from build123d import *

# Parameters (mm, degrees)
SKETCH_1_W                         = 130
SKETCH_1_H                         = 22
ARM_WEB_L130_W22_T6_DEPTH          = 6
SKETCH_2_R                         = 14
SPLIT_CLAMP_HUB_DEPTH              = 12
SKETCH_3_R                         = 16
WRIST_END_R16_DEPTH                = 6
SHAFT_D5P2_AND_WRIST_M3_DEPTH      = 148.363496158
SHAFT_D5P2_AND_WRIST_M3_DEPTH_BACK = 148.363496158
SKETCH_4_R                         = 2.6
SKETCH_4_R_2                       = 1.7
CLAMP_SPLIT_1P2_DEPTH              = 148.363496158
CLAMP_SPLIT_1P2_DEPTH_BACK         = 148.363496158
SKETCH_5_W                         = 1.2
SKETCH_5_H                         = 12.8
CLAMP_CROSSBOLT_M3_DEPTH           = 148.363496158
CLAMP_CROSSBOLT_M3_DEPTH_BACK      = 148.363496158
SKETCH_6_R                         = 1.7


with BuildPart() as part:
    # 草图1 → Arm_web_L130_W22_T6 (new body)
    with BuildSketch(Plane.XY):
        with Locations((65, 0)):
            Rectangle(SKETCH_1_W, SKETCH_1_H)
    extrude(amount=ARM_WEB_L130_W22_T6_DEPTH)

    # 草图2 → Split_clamp_hub (add)
    with BuildSketch(Plane.XY):
        with Locations(Location((0, 0, 0), (0, 0, 308.213210702))):
            Circle(SKETCH_2_R)
    extrude(amount=SPLIT_CLAMP_HUB_DEPTH)

    # 草图3 → Wrist_end_R16 (add)
    with BuildSketch(Plane.XY):
        with Locations((130, 0)):
            Circle(SKETCH_3_R)
    extrude(amount=WRIST_END_R16_DEPTH)

    # 草图4 → Shaft_D5p2_and_wrist_M3 (cut, two sides: drawn at the far end of the back side and taken through both)
    with BuildSketch(Plane.XY.offset(-SHAFT_D5P2_AND_WRIST_M3_DEPTH_BACK)):
        Circle(SKETCH_4_R)
        with Locations((124, 0)):
            Circle(SKETCH_4_R_2)
        with Locations((136, 0)):
            Circle(SKETCH_4_R_2)
    extrude(amount=SHAFT_D5P2_AND_WRIST_M3_DEPTH + SHAFT_D5P2_AND_WRIST_M3_DEPTH_BACK, mode=Mode.SUBTRACT)

    # 草图5 → Clamp_split_1p2 (cut, two sides: drawn at the far end of the back side and taken through both)
    with BuildSketch(Plane.XY.offset(-CLAMP_SPLIT_1P2_DEPTH_BACK)):
        with Locations((0, 8.6)):
            Rectangle(SKETCH_5_W, SKETCH_5_H)
    extrude(amount=CLAMP_SPLIT_1P2_DEPTH + CLAMP_SPLIT_1P2_DEPTH_BACK, mode=Mode.SUBTRACT)

    # 草图6 → Clamp_crossbolt_M3 (cut, two sides: drawn at the far end of the back side and taken through both)
    with BuildSketch(Plane(origin=(0, 0, 0), x_dir=(0, 0, -1), z_dir=(1, 0, 0)).offset(-CLAMP_CROSSBOLT_M3_DEPTH_BACK)):
        with Locations((-8.5, 9)):
            Circle(SKETCH_6_R)
    extrude(amount=CLAMP_CROSSBOLT_M3_DEPTH + CLAMP_CROSSBOLT_M3_DEPTH_BACK, mode=Mode.SUBTRACT)


solid = part.part
CAD build for the part. Positions are in the model's coordinates, mm. A direction names the side the tool comes from. Round coordinates to 2 decimals unless told otherwise and drop trailing zeros. Order: outer loops, then holes, each group sorted by start corner. A loop starts at its lowest first (then second) coordinate and runs counter-clockwise, first axis right, second up. Notation, with made-up numbers: (-1.75, 53.25) - (13.25, 53.25) arc R26 cw to (13.25, 83.25) - close; hole circle Ø10 at (68, 67.25). An arc over 180 degrees is marked (long way). Return JSON: item names as keys, results as strings.
(1) Cut at B-B (x = 136). Give the cut face in (y, z), then the cut area to 3 significant figures.
Answer key:
{"outline": "(-14.83, 0) - (-1.7, 0) - (-1.7, 6) - (-14.83, 6) - close; (1.7, 0) - (14.83, 0) - (14.83, 6) - (1.7, 6) - close", "area": "158 mm^2"}
(2) Tool access for faces 4 (the face through (63, 11, 3)), 5 (the face through (63, -11, 3)), 6 (the face through (-0.1, -2.6, 5.9)): list every direction of +Z, -Z, +X, -X, +Y, -Y with a clear straight run to the whole face (end or side of a thin tool).
Answer key:
{"face 4": "+Z, -Z, +Y", "face 5": "+Z, -Z, -Y", "face 6": "+Z, -Z"}
(3) Pull direction Y, two halves, no side cores. Call faces 1 (the face through (2, -2, 12)), 2 (the face through (137.62, 0.51, 2.96)), 3 (the face through (145.99, -0.53, 2.96)): +Y half, -Y half, draft (parallel to the pull), parting line (faces both ways), or undercut.
Answer key:
{"face 1": "draft", "face 2": "undercut", "face 3": "parting line"}
(4) Cut at A-A (z = 2.5). Give the cut face in (x, y), then the cut area to 3 significant figures.
Answer key:
{"outline": "(-0.6, 2.53) - (-0.6, 13.99) arc R14 ccw (long way) to (8.66, -11) - (118.38, -11) arc R16 ccw (long way) to (118.38, 11) - (8.66, 11) arc R14 ccw to (0.6, 13.99) - (0.6, 2.53) arc R2.6 cw (long way) to start; hole circle Ø3.4 at (124, 0); hole circle Ø3.4 at (136, 0)", "area": "3,630 mm^2"}
(5) Cut at D-D (x = 37.5). Give the cut face in (y, z).
Answer key:
{"outline": "(-11, 0) - (11, 0) - (11, 6) - (-11, 6) - close"}
(6) Wall check: probe 1 along X at (y, z) = (0, 2.9); probe 2 along Z at (x, y) = (-4, 9); probe 3 along Z at (x, y) = (81.5, -2.5). Give the ranges that are in metal, low to high. Write a range as from..to.
Answer key:
{"probe 1": "x = -14..-2.6, 2.6..122.3, 125.7..134.3, 137.7..146", "probe 2": "z = 0..6.8, 10.2..12", "probe 3": "z = 0..6"}
(7) Cut at C-C (y = 9). Give the cut face in (x, z), then the cut area to 3 significant figures.
Answer key:
{"outline": "(-10.72, 0) - (-0.6, 0) - (-0.6, 6.8) - (-10.72, 6.8) - close; (-10.72, 10.2) - (-0.6, 10.2) - (-0.6, 12) - (-10.72, 12) - close; (0.6, 0) - (143.23, 0) - (143.23, 6) - (10.72, 6) - (10.72, 6.8) - (0.6, 6.8) - close; (0.6, 10.2) - (10.72, 10.2) - (10.72, 12) - (0.6, 12) - close", "area": "969 mm^2"}
(8) Pin check, flat tips, straight feed: pin 1 Ø3.5 at (y, z) = (11, 4) entering from -X; pin 2 Ø4 at (y, z) = (9, 8.5) entering from +X; pin 3 Ø4.5 at (x, y) = (124, 0) entering from +Z. Stop position of each tip, or through.
Answer key:
{"pin 1": "stops at x = -10.51", "pin 2": "stops at x = 12.12", "pin 3": "stops at z = 6"}
